Autodesk Inventor part; units mm, degrees
ref_plane "RR_XY" through (0, 0, 0) normal (0, 0, 1) x (1, 0, 0)
ref_plane "RR_YZ" through (0, 0, 0) normal (1, 0, 0) x (0, 1, 0)
ref_plane "RR_ZX" through (0, 0, 0) normal (0, 1, 0) x (0, 0, 1)
sketch "Sketch_1" plane through (0, 0, 0) normal (0, 0, 1) x (1, 0, 0)
  arc A0 (4.042, -4.8974) -> (-4.042, -4.8974) centre (0, 0) ccw
  arc A1 (-4.042, -4.8974) -> (-2.6862, -4.6526) centre (-3.4677, -4.2015) ccw
  line L0 (-2.6862, -4.6526) -> (-1.5816, -2.7394)
  arc A2 (-1.5816, -2.7394) -> (-1.7038, -2.06) centre (-2.0446, -2.472) ccw
  arc A3 (-2.636, -0.4456) -> (-1.7038, -2.06) centre (0, 0) ccw
  arc A4 (-2.636, -0.4456) -> (-3.1632, 0) centre (-3.1632, -0.5347) ccw
  line L1 (-3.1632, 0) -> (-3.8636, 0)
  arc A5 (-4.458, 0.6941) -> (-3.8636, 0) centre (-3.8636, 0.6016) ccw
  arc A6 (-2.8301, 3.5137) -> (-4.458, 0.6941) centre (0, 0) ccw
  arc A7 (-1.9318, 3.3459) -> (-2.8301, 3.5137) centre (-2.4527, 3.0452) ccw
  line L2 (-1.9318, 3.3459) -> (-1.5816, 2.7394)
  arc A8 (-1.5816, 2.7394) -> (-0.9321, 2.5056) centre (-1.1185, 3.0067) ccw
  arc A9 (0.9321, 2.5056) -> (-0.9321, 2.5056) centre (0, 0) ccw
  arc A10 (0.9321, 2.5056) -> (1.5816, 2.7394) centre (1.1185, 3.0067) ccw
  line L3 (1.5816, 2.7394) -> (1.9318, 3.3459)
  arc A11 (2.8301, 3.5137) -> (1.9318, 3.3459) centre (2.4527, 3.0452) ccw
  arc A12 (4.458, 0.6941) -> (2.8301, 3.5137) centre (0, 0) ccw
  arc A13 (3.8636, 0) -> (4.458, 0.6941) centre (3.8636, 0.6016) ccw
  line L4 (3.8636, 0) -> (3.1632, 0)
  arc A14 (3.1632, 0) -> (2.636, -0.4456) centre (3.1632, -0.5347) ccw
  arc A15 (1.7038, -2.06) -> (2.636, -0.4456) centre (0, 0) ccw
  arc A16 (1.7038, -2.06) -> (1.5816, -2.7394) centre (2.0446, -2.472) ccw
  line L5 (1.5816, -2.7394) -> (2.6862, -4.6526)
  arc A17 (2.6862, -4.6526) -> (4.042, -4.8974) centre (3.4677, -4.2015) ccw
extrude "Extrusion1" add sketch "Sketch_1" along normal mid plane 1.1049
ref_plane "RR_XY" through (0, 0, 0) normal (0, 0, 1) x (1, 0, 0)
ref_plane "RR_YZ" through (0, 0, 0) normal (1, 0, 0) x (0, 1, 0)
ref_plane "RR_ZX" through (0, 0, 0) normal (0, 1, 0) x (0, 0, 1)
properties part number "D-5866"
Geometry check sheet. Reference: the model listing, model coordinates, mm. A direction names the side the tool comes from. Coordinates: 2 decimals unless noted, no trailing zeros. Order: outer loops, then holes, each group sorted by start corner. A loop starts at its lowest first (then second) coordinate and runs counter-clockwise, first axis right, second up. Notation, with made-up numbers: M -12.75,1 L 40.25,1 A29 cw 40.25,31 Z; hole C 32,74 d10. An arc over 180 degrees is marked long. One line per question, with ' | ' between items. Start each with the question number.
Item 1: Set-up check for faces 1 (the flat face through (-2.14, -3.71, -0.01)), 2 (the cylindrical face through (2.335, 3.635, -0.008)), 3 (the flat face through (0, 3, -0.552)): record each of +Z, -Z, +X, -X, +Y, -Y from which the full face is reachable in a straight line by a thin tool's end or side.
Item 2: Gauge pin test, flat end, axial feed: pin 1 (6 mm diameter, centred on x = 0.5, y = -3, fed in from +Z). Record the tip position at first contact, or that the pin passes through.
Item 3: Cross-section at D-D on y = -3.75. Enter the section's corners in (x, z), then the cut area to 3 significant figures.
Item 4: Draft check along X on faces 4 (the flat face through (0, 3, 0.552)), 5 (the cylindrical face through (-0.218, 6.346, -0.008)), 6 (the cylindrical face through (2.32, -1.33, -0.01)), 7 (the cylindrical face through (-0.013, 2.673, -0.008)). Enter one of: pulls with the +X half, pulls with the -X half, needs draft (parallel to the pull), parting line crosses it, or undercut.
Item 5: Cross-section at C-C on x = 0. Enter the section's corners in (y, z).
Item 6: Cross-section at A-A on z = 0.1. Enter the section's corners in (x, y), then the cut area to 3 significant figures.
Item 7: Cross-section at B-B on y = -1.25. Enter the section's corners in (x, z).
Item 8: Material ranges on L1, parallel to X at y = -3.75, z = 0.1; L2, parallel to X at y = 0.25, z = 0; L3, parallel to Y at x = 2.75, z = 0.4, recorded low to high. Write a range as [from, to].
Findings:
1) face 1: +Z, -Z, -Y | face 2: +Z, -Z | face 3: -Z, +X, -X, +Y, -Y
2) pin 1: stops at z = 0.55
3) outline: M -5.12,-0.55 L -2.17,-0.55 L -2.17,0.55 L -5.12,0.55 Z; M 2.17,-0.55 L 5.12,-0.55 L 5.12,0.55 L 2.17,0.55 Z | area: 6.54 mm²
4) face 4: needs draft | face 5: parting line crosses it | face 6: undercut | face 7: undercut
5) outline: M 2.67,-0.55 L 6.35,-0.55 L 6.35,0.55 L 2.67,0.55 Z
6) outline: M -4.46,0.69 A4.51 cw -2.83,3.51 A0.6 cw -1.93,3.35 L -1.58,2.74 A0.53 ccw -0.93,2.51 A2.67 cw 0.93,2.51 A0.53 ccw 1.58,2.74 L 1.93,3.35 A0.6 cw 2.83,3.51 A4.51 cw 4.46,0.69 A0.6 cw 3.86,0 L 3.16,0 A0.53 ccw 2.64,-0.45 A2.67 cw 1.7,-2.06 A0.53 ccw 1.58,-2.74 L 2.69,-4.65 A0.9 ccw 4.04,-4.9 A6.35 ccw long -4.04,-4.9 A0.9 ccw -2.69,-4.65 L -1.58,-2.74 A0.53 ccw -1.7,-2.06 A2.67 cw -2.64,-0.45 A0.53 ccw -3.16,0 L -3.86,0 A0.6 cw Z | area: 72.7 mm²
7) outline: M -6.23,-0.55 L -2.36,-0.55 L -2.36,0.55 L -6.23,0.55 Z; M 2.36,-0.55 L 6.23,-0.55 L 6.23,0.55 L 2.36,0.55 Z
8) L1: x = [-5.12, -2.17], [2.17, 5.12] | L2: x = [-6.35, -4.35], [4.35, 6.35] | L3: y = [-4.75, -0.2], [3.57, 5.72]
